Geometry check sheet. Reference: the model listing, model coordinates, mm. A direction names the side the tool comes from. Give positions to 0.01 mm unless a question says otherwise; leave off trailing zeros. Write each loop counter-clockwise with the first axis right and the second up, starting at its lowest first coordinate (ties: lowest second). Pieces come first, ordered by that corner, then holes. Notation, with made-up numbers: (50, 78) -> (101, 78) arc R14 cw to (101, 105) -> close; hole circle Ø6 at (57, 55). An arc over 180 degrees is marked (long way). Write item = value, one per line. Start each with the question number.
1. Set-up check for faces 5 (the flat face through (-2, 3, 2)), 6 (the flat face through (-20, -2, 0)), 7 (the cylindrical face through (-3.905, -2.028, -0.867)): record each of +Z, -Z, +X, -X, +Y, -Y from which the full face is reachable in a straight line by a thin tool's end or side.
2. Mould release check, pull along Z, two halves, no side actions. Record for faces 1 (the cylindrical face through (-3.905, 4.479, -0.867)), 2 (the flat face through (-5, -4, 0)), 3 (the flat face through (0, -2, 5)), 4 (the cylindrical face through (-4.88, 2.96, -1.08)): pulls with the +Z half, pulls with the -Z half, needs draft (parallel to the pull), parting line crosses it, or undercut.
3. Cross-section at D-D, the plane y = 5. Record the cut outline in (x, z).
4. Cross-section at B-B, the plane x = 3. Record the cut outline in (y, z), plus the area to 3 significant figures.
5. Depth check by flat-ended pin: P1, Ø3, axis at x = -8.5, z = -0.5, coming from the +Y side; P2, Ø5, axis at x = 0, z = 0, coming from the +Y side. Enter the tip coordinate at first touch or a pass-through.
6. Cross-section at C-C, the plane z = 3. Record the cut outline in (x, y).
7. Cross-section at A-A, the plane z = 0. Record the cut outline in (x, y).
8. Thickness scan on line 1 along X through (y, z) = (2.2, 0); line 2 along X through (y, z) = (-1.9, 0); line 3 along Y through (x, z) = (-2.5, 2). Record the ranges inside material, lowest first.
```python
from build123d import *

# Parameters (mm, degrees)
SKETCH1_R           = 4
SKETCH1_R_2         = 2.1
BOSS_EXTRUDE1_DEPTH = 3
SKETCH2_R           = 5
SKETCH2_R_2         = 4
BOSS_EXTRUDE2_DEPTH = 6
BOSS_EXTRUDE3_START = -4
SKETCH3_W           = 40
SKETCH3_H           = 10
SKETCH3_R           = 4
BOSS_EXTRUDE3_DEPTH = 4


with BuildPart() as part:
    # Sketch1 → Boss-Extrude1 (new body)
    with BuildSketch(Plane(origin=(0, 0, 0), x_dir=(1, 0, 0), z_dir=(0, 1, 0))):
        with Locations(Location((0, 0, 0), (0, 0, 270))):
            Circle(SKETCH1_R)
        with Locations(Location((0, 0, 0), (0, 0, 270))):
            Circle(SKETCH1_R_2, mode=Mode.SUBTRACT)
    extrude(amount=BOSS_EXTRUDE1_DEPTH)

    # Sketch2 → Boss-Extrude2 (add)
    with BuildSketch(Plane(origin=(0, 0, 0), x_dir=(1, 0, 0), z_dir=(0, 1, 0))):
        with Locations(Location((0, 0, 0), (0, 0, 270))):
            Circle(SKETCH2_R)
        with Locations(Location((0, 0, 0), (0, 0, 270))):
            Circle(SKETCH2_R_2, mode=Mode.SUBTRACT)
    extrude(amount=BOSS_EXTRUDE2_DEPTH)

    # Sketch3 → Boss-Extrude3 (add)
    with BuildSketch(Plane(origin=(0, 0, 0), x_dir=(1, 0, 0), z_dir=(0, 1, 0)).offset(BOSS_EXTRUDE3_START)):
        Rectangle(SKETCH3_W, SKETCH3_H)
        with Locations(Location((0, 0, 0), (0, 0, 270))):
            Circle(SKETCH3_R, mode=Mode.SUBTRACT)
    extrude(amount=BOSS_EXTRUDE3_DEPTH)


solid = part.part
```
Answers:
q1.face_5 = +Y
q1.face_6 = +Z, -Z, -X, +Y, -Y
q1.face_7 = -Y
q2.face_1 = undercut
q2.face_2 = needs draft
q2.face_3 = pulls with the +Z half
q2.face_4 = parting line crosses it
q3.outline = circle Ø10 at (0, 0); hole circle Ø8 at (0, 0)
q4.outline = (-4, -5) -> (0, -5) -> (0, -4) -> (6, -4) -> (6, -2.65) -> (3, -2.65) -> (3, 2.65) -> (6, 2.65) -> (6, 4) -> (0, 4) -> (0, 5) -> (-4, 5) -> (-4, 2.65) -> (0, 2.65) -> (0, -2.65) -> (-4, -2.65) -> close
q4.area = 51.0 mm^2
q5.P1 = 0
q5.P2 = 3
q6.outline = (-20, -4) -> (-2.65, -4) -> (-2.65, 0) -> (2.65, 0) -> (2.65, -4) -> (20, -4) -> (20, 0) -> (4, 0) -> (4, 6) -> (2.65, 6) -> (2.65, 3) -> (-2.65, 3) -> (-2.65, 6) -> (-4, 6) -> (-4, 0) -> (-20, 0) -> close
q7.outline = (-20, -4) -> (-4, -4) -> (-4, 0) -> (-2.1, 0) -> (-2.1, 3) -> (-4, 3) -> (-4, 6) -> (-5, 6) -> (-5, 0) -> (-20, 0) -> close; (2.1, 0) -> (4, 0) -> (4, -4) -> (20, -4) -> (20, 0) -> (5, 0) -> (5, 6) -> (4, 6) -> (4, 3) -> (2.1, 3) -> close
q8.line_1 = -5 to -2.1, 2.1 to 5
q8.line_2 = -20 to -4, 4 to 20
q8.line_3 = 0 to 3
